Answer from the drawing. Dimensions are ordinates in mm from the lowest x, y and z of the part. A direction names the side the tool comes from. Round coordinates to 2 decimals unless told otherwise and drop trailing zeros. Loops run counter-clockwise (first coordinate to the right, second up) from the corner with the lowest first, then second, coordinate; pieces in that order, holes last.
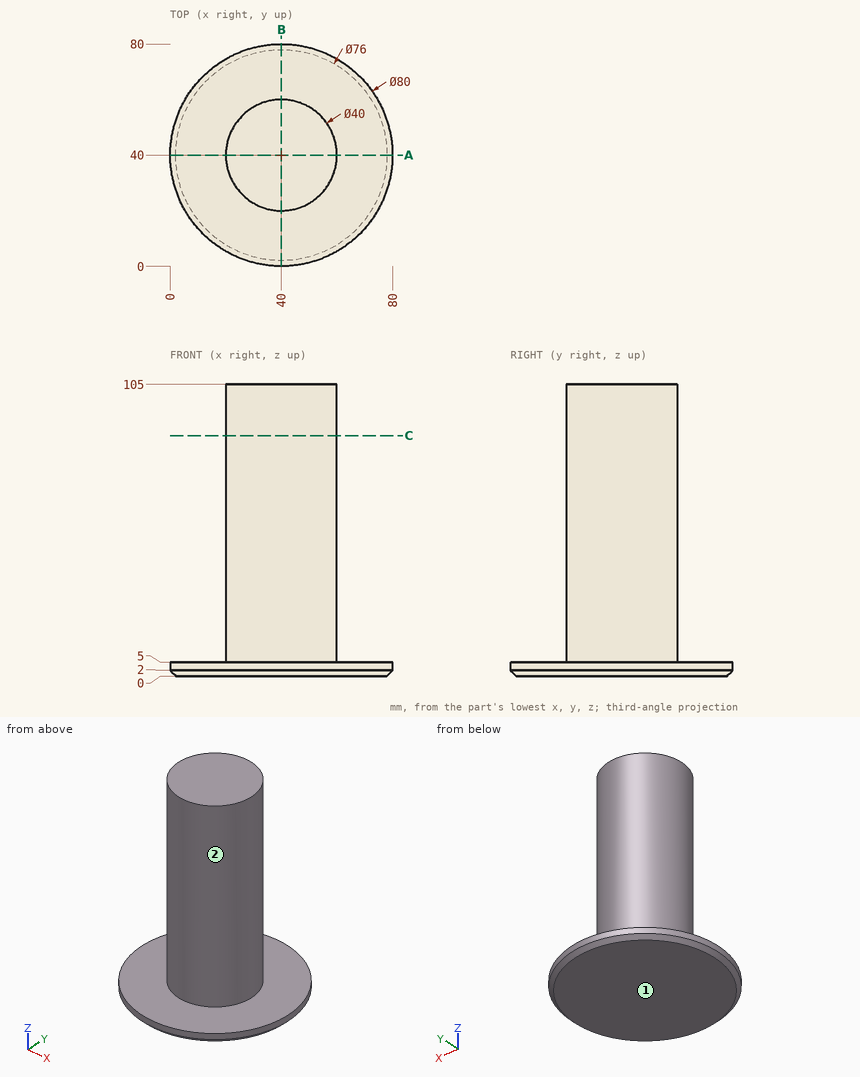
1. Which of the six approach directions +Z, -Z, +X, -X, +Y, -Y give full straight-line access (tool end or side, diameter ignored) to the marked faces 1 and 2?
Answer key:
face 1: -Z, +X, -X, +Y, -Y
face 2: +Z
2. Given pin 1 (1 mm diameter, centred on x = 46, z = 91, fed in from +Y); pin 2 (6 mm diameter, centred on y = 30.5, z = 85.5, fed in from -X); pin 3 (12 mm diameter, centred on y = 63, z = 90.5, fed in from -X), each flat-ended and moving along its own axis, determine where each tip first touches the part or whether it passes through.
Answer key:
pin 1: stops at y = 59.23
pin 2: stops at x = 21.09
pin 3: stops at x = 29.46
3. Find section A-A (y = 40). Write down the section's boundary in (x, z), then the cut area to 3 significant figures.
Answer key:
outline: (0, 2) - (2, 0) - (78, 0) - (80, 2) - (80, 5) - (60, 5) - (60, 105) - (20, 105) - (20, 5) - (0, 5) - close
area: 4,400 mm2
4. Find section C-C (z = 86.5). Write down the section's boundary in (x, y), then the cut area to 3 significant figures.
Answer key:
outline: circle Ø40 at (40, 40)
area: 1,260 mm2
5. Consider probe 1 along Z at (x, y) = (9.5, 30.5); probe 2 along X at (y, z) = (40.5, 56.5); probe 3 along X at (y, z) = (24.5, 46). Determine where each line is inside the solid, lowest interval first.
Answer key:
probe 1: z = 0 to 5
probe 2: x = 20.01 to 59.99
probe 3: x = 27.36 to 52.64
